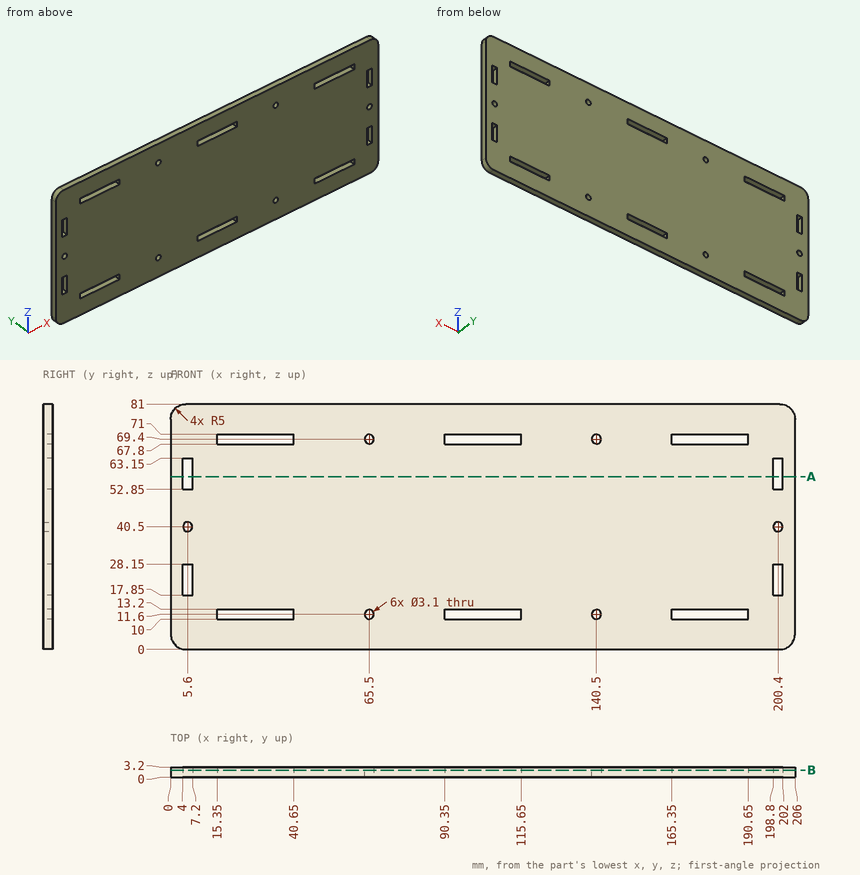
Design review of the part shown in the three views and the two pictorial views. Dimensions are in mm from the part's minimum x, y and z. Give positions to 0.01 mm unless a question says otherwise; leave off trailing zeros. Write each loop counter-clockwise with the first axis right and the second up, starting at its lowest first coordinate (ties: lowest second). Pieces come first, ordered by that corner, then holes. Notation, with made-up numbers: M 78.25,67.25 L 96.25,67.25 A28 ccw 96.25,106.25 Z; hole C 23,66 d9. An arc over 180 degrees is marked long. One line per item, written item: value.
1) For line 1 (Z direction, x = 65.5, y = 1.9); line 2 (Z direction, x = 5.6, y = 0.8); line 3 (Z direction, x = 105.5, y = 1.3), list the stretches that pass through material, from the lowest coordinate up. Write a range as from..to.
Results are:
line 1: z = 0..10.05, 13.15..67.85, 70.95..81
line 2: z = 0..17.85, 28.15..38.95, 42.05..52.85, 63.15..81
line 3: z = 0..10, 13.2..67.8, 71..81
2) Take a section at B-B, the plane y = 2.35. Count the separate pieces of the cut face and the enclosed holes in it, then the cut area to 3 significant figures.
Results are:
separate pieces: 1
enclosed holes: 16
area: 16,000 mm²
3) Take a section at A-A, the plane z = 57. Write out the cut boundary in (x, y).
Results are:
outline: M 0,0 L 4,0 L 4,3.2 L 0,3.2 Z; M 7.2,0 L 198.8,0 L 198.8,3.2 L 7.2,3.2 Z; M 202,0 L 206,0 L 206,3.2 L 202,3.2 Z
